Could you check a few things on this model? Use its own coordinates, in mm. Coordinates: 2 decimals unless noted, no trailing zeros. Write each loop counter-clockwise with the first axis right and the second up, starting at its lowest first coordinate (ties: lowest second). Pieces come first, ordered by that corner, then holes.
Item 1: If I drill on probe 1 along Y at (x, z) = (84, 0.35); probe 2 along Y at (x, z) = (15, 0.35); probe 3 along Y at (x, z) = (-84, 0.75), over which ranges is the centre line in solid material (lowest first)?
Item 2: I want a section at D-D on x = 15. Please give me the cut outline in (y, z).
Item 3: For P1, Ø2.5, axis at x = -84, y = -52, coming from the -Z side; P2, Ø0.5, axis at y = 5.5, z = 0.5, coming from the -X side, each with a flat end and sliding along its axis, tell me the tip position at first contact or that it passes through.
Item 4: I want a section at C-C on y = -52. Please give me the cut outline in (x, z).
Item 5: I want a section at B-B on x = 84. Please give me the cut outline in (y, z).
Item 6: I want a section at A-A on z = 0.3. Please give me the cut outline in (x, y), then the cut area to 3 significant figures.
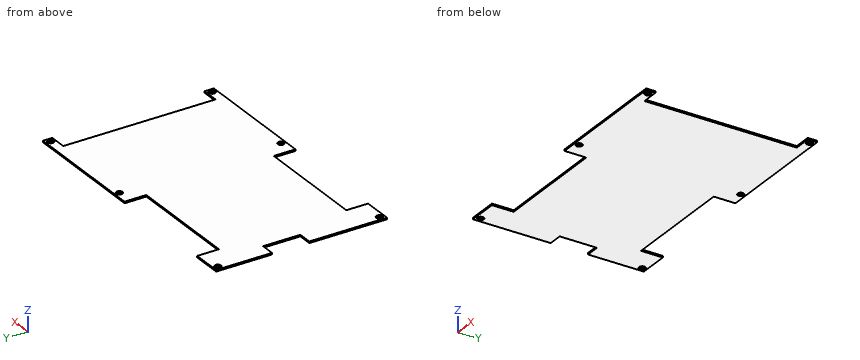
from build123d import *

# Parameters (mm, degrees)
F1_W     = 174
F1_H     = 110
F2_DEPTH = 1
F3_W     = 73
F3_H     = 14
F3_W_2   = 9
F3_H_2   = 24
F3_W_3   = 11
F3_H_3   = 98
F4_DEPTH = 25
F6_D     = 4


with BuildPart() as f2:
    # F1 (on Top) → F2 (new body)
    with BuildSketch(Plane.XY):
        Rectangle(F1_W, F1_H)
    extrude(amount=F2_DEPTH)

    # F3 (on face) → F4 (cut)
    with BuildSketch(Plane.XY.offset(1)):
        with Locations((-31.5, 48)):
            Rectangle(F3_W, F3_H)
        with Locations((-31.5, -48)):
            Rectangle(F3_W, F3_H)
        with Locations((-82.5, 7)):
            Rectangle(F3_W_2, F3_H_2)
        with Locations((81.5, 0)):
            Rectangle(F3_W_3, F3_H_3)
    extrude(amount=-F4_DEPTH, mode=Mode.SUBTRACT)

    # F6 (through all)
    with Locations(Plane.XY.offset(1)):
        with Locations((-84, 52), (15, -52), (15, 52), (84, 52), (84, -52), (-84, -52)):
            Hole(F6_D / 2)


solid = f2.part
Response values:
1. probe 1: y = -55 to -54, -50 to -49, 49 to 50, 54 to 55
1. probe 2: y = -55 to -54, -50 to 50, 54 to 55
1. probe 3: y = -55 to -54, -50 to -5, 19 to 50, 54 to 55
2. outline: (-55, 0) - (-54, 0) - (-54, 1) - (-55, 1) - close; (-50, 0) - (50, 0) - (50, 1) - (-50, 1) - close; (54, 0) - (55, 0) - (55, 1) - (54, 1) - close
3. P1: passes through
3. P2: stops at x = -78
4. outline: (-87, 0) - (-86, 0) - (-86, 1) - (-87, 1) - close; (-82, 0) - (-68, 0) - (-68, 1) - (-82, 1) - close; (5, 0) - (13, 0) - (13, 1) - (5, 1) - close; (17, 0) - (82, 0) - (82, 1) - (17, 1) - close; (86, 0) - (87, 0) - (87, 1) - (86, 1) - close
5. outline: (-55, 0) - (-54, 0) - (-54, 1) - (-55, 1) - close; (-50, 0) - (-49, 0) - (-49, 1) - (-50, 1) - close; (49, 0) - (50, 0) - (50, 1) - (49, 1) - close; (54, 0) - (55, 0) - (55, 1) - (54, 1) - close
6. outline: (-87, -55) - (-68, -55) - (-68, -41) - (5, -41) - (5, -55) - (87, -55) - (87, -49) - (76, -49) - (76, 49) - (87, 49) - (87, 55) - (5, 55) - (5, 41) - (-68, 41) - (-68, 55) - (-87, 55) - (-87, 19) - (-78, 19) - (-78, -5) - (-87, -5) - close; hole circle Ø4 at (-84, -52); hole circle Ø4 at (-84, 52); hole circle Ø4 at (15, -52); hole circle Ø4 at (15, 52); hole circle Ø4 at (84, -52); hole circle Ø4 at (84, 52)
6. area: 15,700 mm2
